Build history of the part. All positions in model axes, mm. Face numbers are marked on the shaded views. Give positions to 0.01 mm unless a question says otherwise; leave off trailing zeros. Loops run counter-clockwise (first coordinate to the right, second up) from the corner with the lowest first, then second, coordinate; pieces in that order, holes last.
1) Wall check: line 1 (X direction, y = 1.5, z = 16); line 2 (Z direction, x = 17, y = 1.6); line 3 (Z direction, x = 16.5, y = 0.3). Give the ranges that are in metal, low to high.
2) Band-saw the part on A-A on x = 16. List the corners of the cut face in (y, z), then the cut area to 3 significant figures.
3) Band-saw the part on B-B on z = 16. List the corners of the cut face in (x, y), then the cut area to 3 significant figures.
4) Flat gauge pin, fed straight in: P1, Ø2.5, axis at x = 28.5, z = 16, coming from the +Y side. Where does the tip first touch, or does it go through?
5) Two-plate mould, pull along Z, no slides. Class the marked faces 1, 2 and 3: +Z half, -Z half, draft (parallel to the pull), parting line (faces both ways), or undercut.
6) Band-saw the part on C-C on y = 0.9. State how many separate pieces and enclosed holes the cut face has, then the cut area to 3 significant figures.
```python
from build123d import *

# Parameters (mm, degrees)
SKETCH1_W           = 32
SKETCH1_H           = 32
BOSS_EXTRUDE1_DEPTH = 4
SKETCH2_R           = 9.15
SKETCH2_R_2         = 1.4
CUT_EXTRUDE1_DEPTH  = 4
FILLET1_SIZE        = 13


with BuildPart() as part:
    # Sketch1 → Boss-Extrude1 (new body)
    with BuildSketch(Plane(origin=(0, 0, 0), x_dir=(1, 0, 0), z_dir=(0, 1, 0))):
        with Locations((16, -16)):
            Rectangle(SKETCH1_W, SKETCH1_H)
    extrude(amount=BOSS_EXTRUDE1_DEPTH)

    # Sketch2 → Cut-Extrude1 (cut)
    with BuildSketch(Plane(origin=(0, 0, 0), x_dir=(-1, 0, 0), z_dir=(0, -1, 0))):
        with Locations(Location((-16, -16, 0), (0, 0, 90))):
            Circle(SKETCH2_R)
        with Locations(Location((-16, -28.5, 0), (0, 0, 90))):
            Circle(SKETCH2_R_2)
        with Locations(Location((-28.5, -16, 0), (0, 0, 90))):
            Circle(SKETCH2_R_2)
        with Locations(Location((-16, -3.5, 0), (0, 0, 90))):
            Circle(SKETCH2_R_2)
        with Locations(Location((-3.5, -16, 0), (0, 0, 90))):
            Circle(SKETCH2_R_2)
    extrude(amount=-CUT_EXTRUDE1_DEPTH, mode=Mode.SUBTRACT)

    # Fillet1
    # a fillet whose section is not a circle: 13 mm, written as the material it takes off along each edge
    with BuildSketch(Plane(origin=(0, -32.5, 0), x_dir=(1, 0, 0), z_dir=(0, 1, 0)), Plane(origin=(0, -32.5, 32), x_dir=(0, 0, -1), z_dir=(0, 1, 0))) as fillet1_piece_1:
        with BuildLine():
            Bezier((FILLET1_SIZE, 0), (0, 0), (0, -FILLET1_SIZE), weights=[1, 0.333333333, 1])
            Line((0, -FILLET1_SIZE), (0, 0))
            Line((0, 0), (FILLET1_SIZE, 0))
        make_face()
    extrude(amount=69, mode=Mode.SUBTRACT)
    with BuildSketch(Plane(origin=(32, -32.5, 0), x_dir=(-1, 0, 0), z_dir=(0, 1, 0)), Plane(origin=(32, -32.5, 32), x_dir=(0, 0, -1), z_dir=(0, 1, 0))) as fillet1_piece_2:
        with BuildLine():
            Bezier((FILLET1_SIZE, 0), (0, 0), (0, FILLET1_SIZE), weights=[1, 0.333333333, 1])
            Line((0, FILLET1_SIZE), (0, 0))
            Line((0, 0), (FILLET1_SIZE, 0))
        make_face()
    extrude(amount=69, mode=Mode.SUBTRACT)


solid = part.part
```
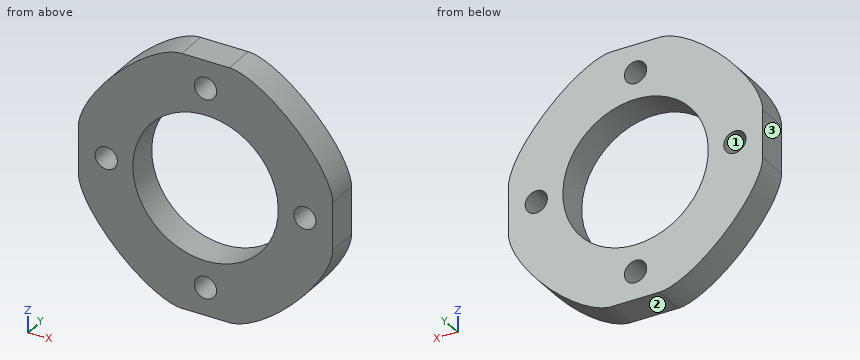
Findings below:
1. line 1: x = 0 to 2.1, 4.9 to 6.85, 25.15 to 27.1, 29.9 to 32
1. line 2: z = 0 to 2.52, 4.48 to 6.9, 25.1 to 27.52, 29.48 to 32
1. line 3: z = 0 to 2.19, 4.81 to 6.86, 25.14 to 27.19, 29.81 to 32
2. outline: (0, 0) - (4, 0) - (4, 2.1) - (0, 2.1) - close; (0, 4.9) - (4, 4.9) - (4, 6.85) - (0, 6.85) - close; (0, 25.15) - (4, 25.15) - (4, 27.1) - (0, 27.1) - close; (0, 29.9) - (4, 29.9) - (4, 32) - (0, 32) - close
2. area: 32.4 mm2
3. outline: (0, 0) - (2.1, 0) - (2.1, 4) - (0, 4) - close; (4.9, 0) - (6.85, 0) - (6.85, 4) - (4.9, 4) - close; (25.15, 0) - (27.1, 0) - (27.1, 4) - (25.15, 4) - close; (29.9, 0) - (32, 0) - (32, 4) - (29.9, 4) - close
3. area: 32.4 mm2
4. P1: passes through
5. face 1: undercut
5. face 2: -Z half
5. face 3: draft
6. separate pieces: 1
6. enclosed holes: 5
6. area: 522 mm2
